Source: CAD feature listing. Evaluate the final solid. Frame: model axes, mm. A direction names the side the tool comes from. Give positions to 0.01 mm unless a question says otherwise; leave off trailing zeros. Order: outer loops, then holes, each group sorted by start corner. A loop starts at its lowest first (then second) coordinate and runs counter-clockwise, first axis right, second up. Notation, with made-up numbers: M -12.5,28.25 L 9.5,28.25 A33 ccw 9.5,65.25 Z; hole C 54.25,87 d8. An arc over 180 degrees is marked long. Answer in a Markdown table with one row per item. Add a question column.
(1) Set-up query: faces 4 (the face through (-123, 5, 100)), 5 (the face through (123, 5, 100)), 6 (the face through (-82.75, 5, 96)). Return all of +Z, -Z, +X, -X, +Y, -Y with unobstructed straight access to the full face (end or side cutting, diameter ignored); none if empty.
(2) Section query A-A, the plane x = 65. Return loops of the section in (y, z).
(3) Section query D-D, the plane y = 6.5. Count the separate pieces of the cut face and the enclosed holes in it, plus the area to 3 significant figures.
(4) Material intervals for line 1 along X through (y, z) = (8.25, -65); line 2 along X through (y, z) = (1.25, 88.5) (3 decimals); line 3 along Z through (x, y) = (-14, 3.75), sorted ascending.
(5) Section query C-C, the plane x = -32.5. Return loops of the section in (y, z), plus the area to 3 significant figures.
(6) Section query B-B, the plane z = 0. Return loops of the section in (x, y).
(7) Pin query (flat end, axial travel): P1, Ø12, axis at x = -61, z = 73, coming from the -Y side; P2, Ø4, axis at x = 47.5, y = 5.5, coming from the -Z side; P3, Ø1.5, axis at x = 88, y = 5, coming from the +Z side; P4, Ø4, axis at y = 6.5, z = 104, coming from the -X side. Return the tip coordinate at first contact, or that it passes through.
(8) Mould query, pull axis Z, two halves, no side actions, for faces 1 (the face through (-80, 5, 100)), 2 (the face through (90, 5, -100)), 3 (the face through (-67.419, 4.93, -68.794)). Classes: pulls with the +Z half, pulls with the -Z half, needs draft (parallel to the pull), parting line crosses it, or undercut.
from build123d import *

# Parameters (mm, degrees)
SKETCH1_W            = 260
SKETCH1_H            = 200
EXTRUDE1_DEPTH       = 10
M4_CLEARANCE_HOLE1_D = 4.5
SKETCH7_W            = 20
SKETCH7_H            = 10
EXTRUDE4_DEPTH       = 10
LPATTERN1_COUNT      = 2
LPATTERN1_PITCH      = 170
LPATTERN1_COUNT_DIR2 = 2
LPATTERN1_PITCH_DIR2 = 210
EXTRUDE5_DEPTH       = 10
MIRROR5_COPY_1_DEPTH = 10
EXTRUDE6_DEPTH       = 10
MIRROR7_COPY_1_DEPTH = 10
SKETCH10_R           = 11.5
EXTRUDE7_DEPTH       = 10
M8_CLEARANCE_HOLE1_D = 9


with BuildPart() as part:
    # Sketch1 → Extrude1 (new body)
    with BuildSketch(Plane(origin=(0, 0, 0), x_dir=(1, 0, 0), z_dir=(0, 1, 0))):
        Rectangle(SKETCH1_W, SKETCH1_H)
    extrude(amount=EXTRUDE1_DEPTH)

    # M4 Clearance Hole1 (through all)
    with Locations(Plane(origin=(0, 10, 0), x_dir=(1, 0, 0), z_dir=(0, 1, 0))):
        with Locations((-85, 45), (85, 45)):
            Hole(M4_CLEARANCE_HOLE1_D / 2)

    # Sketch7 → Extrude4 (add)
    with BuildSketch(Plane(origin=(0, 10, 0), x_dir=(1, 0, 0), z_dir=(0, 1, 0))):
        with Locations((-105, -105)):
            Rectangle(SKETCH7_W, SKETCH7_H)
        with Locations((-65, -105)):
            Rectangle(SKETCH7_W, SKETCH7_H)
    extrude4 = extrude(amount=-EXTRUDE4_DEPTH)

    # LPattern1: Extrude4 2 × 2
    with Locations(*[(i * LPATTERN1_PITCH, 0, -j * LPATTERN1_PITCH_DIR2) for i in range(LPATTERN1_COUNT) for j in range(LPATTERN1_COUNT_DIR2) if (i, j) != (0, 0)]):
        add(extrude4)

    # Sketch8 → Extrude5 (cut)
    with BuildSketch(Plane(origin=(0, 10, 0), x_dir=(1, 0, 0), z_dir=(0, 1, 0))):
        with BuildLine():
            Line((-116.5, -100), (-115, -100))
            Line((-115, -100), (-115, -101.5))
            ThreePointArc((-115, -101.5), (-113.939339828, -98.939339828), (-116.5, -100))
        make_face()
        with BuildLine():
            Line((-95, -101.5), (-95, -100))
            Line((-95, -100), (-93.5, -100))
            ThreePointArc((-93.5, -100), (-96.060660172, -98.939339828), (-95, -101.5))
        make_face()
        with BuildLine():
            Line((-75, -100), (-75, -101.5))
            ThreePointArc((-75, -101.5), (-73.939339828, -98.939339828), (-76.5, -100))
            Line((-76.5, -100), (-75, -100))
        make_face()
        with BuildLine():
            Line((-55, -101.5), (-55, -100))
            Line((-55, -100), (-53.5, -100))
            ThreePointArc((-53.5, -100), (-56.060660172, -98.939339828), (-55, -101.5))
        make_face()
    extrude5 = extrude(amount=-EXTRUDE5_DEPTH, mode=Mode.SUBTRACT)

    # Mirror4: Extrude5 across plane
    add(extrude5.mirror(Plane(origin=(0, 0, 0), x_dir=(0, 0, 1), z_dir=(1, 0, 0))), mode=Mode.SUBTRACT)

    # Mirror5: Extrude5 across plane
    add(extrude5.mirror(Plane.XY), mode=Mode.SUBTRACT)

    # Mirror5 copy 1 sketch → Mirror5 copy 1 (cut)
    with BuildSketch(Plane(origin=(0, 10, 0), x_dir=(-1, 0, 0), z_dir=(0, 1, 0))):
        with BuildLine():
            Line((-116.5, -100), (-115, -100))
            Line((-115, -100), (-115, -101.5))
            ThreePointArc((-115, -101.5), (-113.939339828, -98.939339828), (-116.5, -100))
        make_face()
        with BuildLine():
            Line((-95, -101.5), (-95, -100))
            Line((-95, -100), (-93.5, -100))
            ThreePointArc((-93.5, -100), (-96.060660172, -98.939339828), (-95, -101.5))
        make_face()
        with BuildLine():
            Line((-75, -100), (-75, -101.5))
            ThreePointArc((-75, -101.5), (-73.939339828, -98.939339828), (-76.5, -100))
            Line((-76.5, -100), (-75, -100))
        make_face()
        with BuildLine():
            Line((-55, -101.5), (-55, -100))
            Line((-55, -100), (-53.5, -100))
            ThreePointArc((-53.5, -100), (-56.060660172, -98.939339828), (-55, -101.5))
        make_face()
    extrude(amount=-MIRROR5_COPY_1_DEPTH, mode=Mode.SUBTRACT)

    # Sketch9 → Extrude6 (cut)
    with BuildSketch(Plane(origin=(0, 10, 0), x_dir=(1, 0, 0), z_dir=(0, 1, 0))):
        Polygon((-87.25, -100), (-87.25, -92), (-88.625, -92), (-88.625, -88.3), (-87.25, -88.3), (-87.25, -84), (-82.75, -84), (-82.75, -88.3), (-81.375, -88.3), (-81.375, -92), (-82.75, -92), (-82.75, -100), align=None)
    extrude6 = extrude(amount=-EXTRUDE6_DEPTH, mode=Mode.SUBTRACT)

    # Mirror6: Extrude6 across plane
    add(extrude6.mirror(Plane(origin=(0, 0, 0), x_dir=(0, 0, 1), z_dir=(1, 0, 0))), mode=Mode.SUBTRACT)

    # Mirror7: Extrude6 across plane
    add(extrude6.mirror(Plane.XY), mode=Mode.SUBTRACT)

    # Mirror7 copy 1 sketch → Mirror7 copy 1 (cut)
    with BuildSketch(Plane(origin=(0, 10, 0), x_dir=(-1, 0, 0), z_dir=(0, 1, 0))):
        Polygon((-87.25, -100), (-87.25, -92), (-88.625, -92), (-88.625, -88.3), (-87.25, -88.3), (-87.25, -84), (-82.75, -84), (-82.75, -88.3), (-81.375, -88.3), (-81.375, -92), (-82.75, -92), (-82.75, -100), align=None)
    extrude(amount=-MIRROR7_COPY_1_DEPTH, mode=Mode.SUBTRACT)

    # Sketch10 → Extrude7 (cut)
    with BuildSketch(Plane(origin=(0, 10, 0), x_dir=(1, 0, 0), z_dir=(0, 1, 0))):
        with Locations(Location((-32.5, 0, 0), (0, 0, 270))):
            Circle(SKETCH10_R)
        with Locations(Location((32.5, 0, 0), (0, 0, 270))):
            Circle(SKETCH10_R)
    extrude(amount=-EXTRUDE7_DEPTH, mode=Mode.SUBTRACT)

    # M8 Clearance Hole1 (through all)
    with Locations(Plane(origin=(0, 10, 0), x_dir=(1, 0, 0), z_dir=(0, 1, 0))):
        with Locations((-65, 65), (65, 65), (65, -65), (-65, -65)):
            Hole(M8_CLEARANCE_HOLE1_D / 2)


solid = part.part
Values follow:
| question | item | result |
|---|---|---|
| 1 | face 4 | +Z, -X, +Y, -Y |
| 1 | face 5 | +Z, +X, +Y, -Y |
| 1 | face 6 | +Z, +Y, -Y |
| 2 | outline | M 0,-110 L 10,-110 L 10,-69.5 L 0,-69.5 Z; M 0,-60.5 L 10,-60.5 L 10,60.5 L 0,60.5 Z; M 0,69.5 L 10,69.5 L 10,110 L 0,110 Z |
| 3 | separate pieces | 1 |
| 3 | enclosed holes | 8 |
| 3 | area | 52,100 mm² |
| 4 | line 1 | x = -130 to -69.5, -60.5 to 60.5, 69.5 to 130 |
| 4 | line 2 | x = -130 to -88.625, -81.375 to 81.375, 88.625 to 130 |
| 4 | line 3 | z = -100 to 100 |
| 5 | outline | M 0,-100 L 10,-100 L 10,-11.5 L 0,-11.5 Z; M 0,11.5 L 10,11.5 L 10,100 L 0,100 Z |
| 5 | area | 1,770 mm² |
| 6 | outline | M -130,0 L -44,0 L -44,10 L -130,10 Z; M -21,0 L 21,0 L 21,10 L -21,10 Z; M 44,0 L 130,0 L 130,10 L 44,10 Z |
| 7 | P1 | stops at y = 0 |
| 7 | P2 | stops at z = -100 |
| 7 | P3 | stops at z = 100 |
| 7 | P4 | stops at x = -115 |
| 8 | face 1 | pulls with the +Z half |
| 8 | face 2 | pulls with the -Z half |
| 8 | face 3 | undercut |
